Autodesk Inventor part; units mm, degrees
ref_plane "YZ Plane" through (0, 0, 0) normal (1, 0, 0) x (0, 1, 0)
ref_plane "XZ Plane" through (0, 0, 0) normal (0, 1, 0) x (-1, 0, 0)
ref_plane "XY Plane" through (0, 0, 0) normal (0, 0, 1) x (1, 0, 0)
sketch "Sketch1" plane through (0, 0, 0) normal (0, 0, 1) x (1, 0, 0)
  line L0 (0, 0) -> (0, 7.1437)
  line L1 (0, 7.1437) -> (6.35, 7.1438)
  line L2 (6.35, 7.1438) -> (6.35, 4.7625)
  line L3 (6.35, 4.7625) -> (69.85, 4.7625)
  line L4 (69.85, 4.7625) -> (69.85, 3.9688)
  line L5 (69.85, 3.9688) -> (82.55, 3.9688)
  line L6 (82.55, 3.9688) -> (82.55, 0)
  line L7 (82.55, 0) -> (0, 0)
  dimension "d0" = 7.1437
  dimension "d1" = 4.7625
  dimension "d2" = 3.9688
  dimension "d3" = 6.35
  dimension "d4" = 63.5
  dimension "d5" = 12.7
revolve "Revolution1" add sketch "Sketch1" angle 360 about axis through (82.55, 0, 0) along (-1, 0, 0)
fillet "Fillet1" radius 0.508 2 edges at (0, -7.1437, 0) (6.35, -7.1437, 0)
thread "Thread1"
sketch "Sketch2" plane through (0, 0, 0) normal (-1, 0, 0) x (0, 0, 1)
  circle A0 centre (0, 0) radius 6.6357
  line L0 (0, 2.7496) -> (2.3812, 1.3748)
  line L1 (2.3812, 1.3748) -> (2.3812, -1.3748)
  line L2 (2.3812, -1.3748) -> (0, -2.7496)
  line L3 (0, -2.7496) -> (-2.3813, -1.3748)
  line L4 (-2.3813, -1.3748) -> (-2.3813, 1.3748)
  line L5 (-2.3813, 1.3748) -> (0, 2.7496)
  dimension "d10" = 4.7625
extrude "Extrusion1" cut sketch "Sketch2" against normal blind 3.175 contours L0 L1 L2 L3 L4 L5
properties part number "HW-00065"
The listing builds one solid part. Answer for the finished solid, in the listing's coordinates (mm). A direction names the side the tool comes from. Round coordinates to 2 decimals unless told otherwise and drop trailing zeros. Loops run counter-clockwise (first coordinate to the right, second up) from the corner with the lowest first, then second, coordinate; pieces in that order, holes last.
1) Consider line 1 (X direction, y = -5.5, z = -1.75); line 2 (X direction, y = -4.5, z = 0.25); line 3 (Y direction, x = 41.5, z = 0.25). Determine where each line is inside the solid, lowest interval first.
Outcome:
line 1: x = 0 to 6.35
line 2: x = 0 to 69.85
line 3: y = -4.76 to 4.76
2) For faces 5 (the face through (76.289, 3.666, -1.52)), 6 (the face through (2, 0, 2.381)), 7 (the face through (82.55, 0, 0)), determine the directions among +Z, -Z, +X, -X, +Y, -Y from which every point of the face is accessible in a straight line to the end or side of a thin tool.
Outcome:
face 5: +X
face 6: -X
face 7: +Z, -Z, +X, +Y, -Y
3) Given P1, Ø1.4, axis at y = -1, z = -0.5, coming from the -X side (3 decimals); P2, Ø4, axis at x = 44.5, y = 5, coming from the -Z side; P3, Ø5, axis at x = 16.5, y = -4, coming from the +Z side, each flat-ended and moving along its own axis, determine where each tip first touches the part or whether it passes through.
Outcome:
P1: stops at x = 3.175
P2: stops at z = -3.7
P3: stops at z = 4.52
4) For a pull along Y with two mould halves and no side action, classify faces 1 (the face through (3.212, 6.814, 2.146)), 2 (the face through (0, 0, 3)), 3 (the face through (1.565, -2.072, -1.174)), 4 (the face through (1.565, 2.072, 1.174)) as released by +Y, released by -Y, zero draft, split by the parting line, or undercut.
Outcome:
face 1: split by the parting line
face 2: zero draft
face 3: undercut
face 4: undercut
5) A cutting plane is placed at B-B on x = 53.5. Determine the outline of the cut face in (y, z) (1 decimal), plus the area to 3 significant figures.
Outcome:
outline: circle Ø9.5 at (0, 0)
area: 71.3 mm2
